```python
from build123d import *

# Parameters (mm, degrees)
SKIZZE1_R                       = 32
SKIZZE1_R_2                     = 22
AUFSATZ_LINEAR_AUSTRAGEN1_DEPTH = 6
SKIZZE4_R                       = 30
SCHNITT_LINEAR_AUSTRAGEN1_DEPTH = 0.1
CUT_EXTRUDE_1_DEPTH             = 264.069580964
DURCHGANGSLOCH_F_R_M41_D        = 4.5
F_5_0_5_DURCHMESSER_BOHRUNG1_D  = 5


with BuildPart() as part:
    # Skizze1 → Aufsatz-Linear austragen1 (new body)
    with BuildSketch(Plane.XY):
        with BuildLine():
            Line((84, 49.943328262), (-234, 49.943328262))
            Line((-234, 49.943328262), (-234, -120.056671738))
            Line((-234, -120.056671738), (-183, -120.056671738))
            Line((-183, -120.056671738), (-183, -118.056671738))
            ThreePointArc((-183, -118.056671738), (-182.414213562, -116.642458175), (-181, -116.056671738))
            Line((-181, -116.056671738), (-170, -116.056671738))
            ThreePointArc((-170, -116.056671738), (-168.585786438, -116.642458175), (-168, -118.056671738))
            Line((-168, -118.056671738), (-168, -120.056671738))
            Line((-168, -120.056671738), (-82.5, -120.056671738))
            Line((-82.5, -120.056671738), (-82.5, -118.056671738))
            ThreePointArc((-82.5, -118.056671738), (-81.914213562, -116.642458175), (-80.5, -116.056671738))
            Line((-80.5, -116.056671738), (-69.5, -116.056671738))
            ThreePointArc((-69.5, -116.056671738), (-68.085786438, -116.642458175), (-67.5, -118.056671738))
            Line((-67.5, -118.056671738), (-67.5, -120.056671738))
            Line((-67.5, -120.056671738), (18, -120.056671738))
            Line((18, -120.056671738), (18, -118.056671738))
            ThreePointArc((18, -118.056671738), (18.585786438, -116.642458175), (20, -116.056671738))
            Line((20, -116.056671738), (31, -116.056671738))
            ThreePointArc((31, -116.056671738), (32.414213562, -116.642458175), (33, -118.056671738))
            Line((33, -118.056671738), (33, -120.056671738))
            Line((33, -120.056671738), (84, -120.056671738))
            Line((84, -120.056671738), (84, 49.943328262))
        make_face()
        with BuildLine():
            Line((-143, -112.556671738), (-103, -112.556671738))
            ThreePointArc((-103, -112.556671738), (-100.5, -115.056671738), (-103, -117.556671738))
            Line((-103, -117.556671738), (-143, -117.556671738))
            ThreePointArc((-143, -117.556671738), (-145.5, -115.056671738), (-143, -112.556671738))
        make_face(mode=Mode.SUBTRACT)
        with BuildLine():
            Line((-7, -117.556671738), (-47, -117.556671738))
            ThreePointArc((-47, -117.556671738), (-49.5, -115.056671738), (-47, -112.556671738))
            Line((-47, -112.556671738), (-7, -112.556671738))
            ThreePointArc((-7, -112.556671738), (-4.5, -115.056671738), (-7, -117.556671738))
        make_face(mode=Mode.SUBTRACT)
        with Locations((-185, -0.056671738)):
            Circle(SKIZZE1_R, mode=Mode.SUBTRACT)
        with Locations((-75, -0.056671738)):
            Circle(SKIZZE1_R_2, mode=Mode.SUBTRACT)
        with Locations((35, -0.056671738)):
            Circle(SKIZZE1_R, mode=Mode.SUBTRACT)
    extrude(amount=AUFSATZ_LINEAR_AUSTRAGEN1_DEPTH)

    # Skizze4 → Schnitt-Linear austragen1 (cut)
    # profile 1 of 2: a face of its own
    with BuildSketch(Plane.XY.offset(6)):
        with BuildLine():
            Line((66, -37.056671738), (4, -37.056671738))
            ThreePointArc((4, -37.056671738), (-0.242640687, -35.299312425), (-2, -31.056671738))
            Line((-2, -31.056671738), (-2, 30.943328262))
            ThreePointArc((-2, 30.943328262), (-0.242640687, 35.185968949), (4, 36.943328262))
            Line((4, 36.943328262), (35, 36.943328262))
            Line((35, 36.943328262), (66, 36.943328262))
            ThreePointArc((66, 36.943328262), (70.242640687, 35.185968949), (72, 30.943328262))
            Line((72, 30.943328262), (72, -31.056671738))
            ThreePointArc((72, -31.056671738), (70.242640687, -35.299312425), (66, -37.056671738))
        make_face()
        with Locations((35, -0.056671738)):
            Circle(SKIZZE4_R, mode=Mode.SUBTRACT)
        with BuildLine():
            Line((64, 22.943328262), (60, 22.943328262))
            ThreePointArc((60, 22.943328262), (57, 25.943328262), (60, 28.943328262))
            Line((60, 28.943328262), (64, 28.943328262))
            ThreePointArc((64, 28.943328262), (67, 25.943328262), (64, 22.943328262))
        make_face(mode=Mode.SUBTRACT)
        with BuildLine():
            Line((10, 28.943328262), (6, 28.943328262))
            ThreePointArc((6, 28.943328262), (3, 25.943328262), (6, 22.943328262))
            Line((6, 22.943328262), (10, 22.943328262))
            ThreePointArc((10, 22.943328262), (13, 25.943328262), (10, 28.943328262))
        make_face(mode=Mode.SUBTRACT)
        with BuildLine():
            Line((10, -29.056671738), (6, -29.056671738))
            ThreePointArc((6, -29.056671738), (3, -26.056671738), (6, -23.056671738))
            Line((6, -23.056671738), (10, -23.056671738))
            ThreePointArc((10, -23.056671738), (13, -26.056671738), (10, -29.056671738))
        make_face(mode=Mode.SUBTRACT)
        with BuildLine():
            Line((60, -29.056671738), (64, -29.056671738))
            ThreePointArc((64, -29.056671738), (67, -26.056671738), (64, -23.056671738))
            Line((64, -23.056671738), (60, -23.056671738))
            ThreePointArc((60, -23.056671738), (57, -26.056671738), (60, -29.056671738))
        make_face(mode=Mode.SUBTRACT)
    # profile 2 of 2: a face of its own
    with BuildSketch(Plane.XY.offset(6)):
        with BuildLine():
            Line((-185, 36.943328262), (-216, 36.943328262))
            ThreePointArc((-216, 36.943328262), (-220.242640687, 35.185968949), (-222, 30.943328262))
            Line((-222, 30.943328262), (-222, -31.056671738))
            ThreePointArc((-222, -31.056671738), (-220.242640687, -35.299312425), (-216, -37.056671738))
            Line((-216, -37.056671738), (-154, -37.056671738))
            ThreePointArc((-154, -37.056671738), (-149.757359313, -35.299312425), (-148, -31.056671738))
            Line((-148, -31.056671738), (-148, 30.943328262))
            ThreePointArc((-148, 30.943328262), (-149.757359313, 35.185968949), (-154, 36.943328262))
            Line((-154, 36.943328262), (-185, 36.943328262))
        make_face()
        with Locations((-185, -0.056671738)):
            Circle(SKIZZE4_R, mode=Mode.SUBTRACT)
        with BuildLine():
            Line((-214, -23.056671738), (-210, -23.056671738))
            ThreePointArc((-210, -23.056671738), (-207, -26.056671738), (-210, -29.056671738))
            Line((-210, -29.056671738), (-214, -29.056671738))
            ThreePointArc((-214, -29.056671738), (-217, -26.056671738), (-214, -23.056671738))
        make_face(mode=Mode.SUBTRACT)
        with BuildLine():
            Line((-210, 28.943328262), (-214, 28.943328262))
            ThreePointArc((-214, 28.943328262), (-217, 25.943328262), (-214, 22.943328262))
            Line((-214, 22.943328262), (-210, 22.943328262))
            ThreePointArc((-210, 22.943328262), (-207, 25.943328262), (-210, 28.943328262))
        make_face(mode=Mode.SUBTRACT)
        with BuildLine():
            Line((-156, -23.056671738), (-160, -23.056671738))
            ThreePointArc((-160, -23.056671738), (-163, -26.056671738), (-160, -29.056671738))
            Line((-160, -29.056671738), (-156, -29.056671738))
            ThreePointArc((-156, -29.056671738), (-153, -26.056671738), (-156, -23.056671738))
        make_face(mode=Mode.SUBTRACT)
        with BuildLine():
            Line((-156, 22.943328262), (-160, 22.943328262))
            ThreePointArc((-160, 22.943328262), (-163, 25.943328262), (-160, 28.943328262))
            Line((-160, 28.943328262), (-156, 28.943328262))
            ThreePointArc((-156, 28.943328262), (-153, 25.943328262), (-156, 22.943328262))
        make_face(mode=Mode.SUBTRACT)
    extrude(amount=-SCHNITT_LINEAR_AUSTRAGEN1_DEPTH, mode=Mode.SUBTRACT)

    # Эскиз2 → Вырез-Вытянуть1 (cut, through all)
    with BuildSketch(Plane.XY.offset(6)):
        with BuildLine():
            Line((-214, -29.056671738), (-210, -29.056671738))
            ThreePointArc((-210, -29.056671738), (-207, -26.056671738), (-210, -23.056671738))
            Line((-210, -23.056671738), (-214, -23.056671738))
            ThreePointArc((-214, -23.056671738), (-217, -26.056671738), (-214, -29.056671738))
        make_face()
        with BuildLine():
            Line((-160, -29.056671738), (-156, -29.056671738))
            ThreePointArc((-156, -29.056671738), (-153, -26.056671738), (-156, -23.056671738))
            Line((-156, -23.056671738), (-160, -23.056671738))
            ThreePointArc((-160, -23.056671738), (-163, -26.056671738), (-160, -29.056671738))
        make_face()
        with BuildLine():
            Line((-156, 28.943328262), (-160, 28.943328262))
            ThreePointArc((-160, 28.943328262), (-163, 25.943328262), (-160, 22.943328262))
            Line((-160, 22.943328262), (-156, 22.943328262))
            ThreePointArc((-156, 22.943328262), (-153, 25.943328262), (-156, 28.943328262))
        make_face()
        with BuildLine():
            Line((-214, 22.943328262), (-210, 22.943328262))
            ThreePointArc((-210, 22.943328262), (-207, 25.943328262), (-210, 28.943328262))
            Line((-210, 28.943328262), (-214, 28.943328262))
            ThreePointArc((-214, 28.943328262), (-217, 25.943328262), (-214, 22.943328262))
        make_face()
        with BuildLine():
            Line((6, 22.943328262), (10, 22.943328262))
            ThreePointArc((10, 22.943328262), (13, 25.943328262), (10, 28.943328262))
            Line((10, 28.943328262), (6, 28.943328262))
            ThreePointArc((6, 28.943328262), (3, 25.943328262), (6, 22.943328262))
        make_face()
        with BuildLine():
            Line((64, 28.943328262), (60, 28.943328262))
            ThreePointArc((60, 28.943328262), (57, 25.943328262), (60, 22.943328262))
            Line((60, 22.943328262), (64, 22.943328262))
            ThreePointArc((64, 22.943328262), (67, 25.943328262), (64, 28.943328262))
        make_face()
        with BuildLine():
            Line((64, -23.056671738), (60, -23.056671738))
            ThreePointArc((60, -23.056671738), (57, -26.056671738), (60, -29.056671738))
            Line((60, -29.056671738), (64, -29.056671738))
            ThreePointArc((64, -29.056671738), (67, -26.056671738), (64, -23.056671738))
        make_face()
        with BuildLine():
            Line((10, -23.056671738), (6, -23.056671738))
            ThreePointArc((6, -23.056671738), (3, -26.056671738), (6, -29.056671738))
            Line((6, -29.056671738), (10, -29.056671738))
            ThreePointArc((10, -29.056671738), (13, -26.056671738), (10, -23.056671738))
        make_face()
    extrude(amount=-CUT_EXTRUDE_1_DEPTH, mode=Mode.SUBTRACT)

    # Durchgangsloch für M41 (through all)
    with Locations(Plane(origin=(0, 0, 0), x_dir=(-1, 0, 0), z_dir=(0, 0, -1))):
        with Locations((75, 28.943328262), (95.506096654, 20.449424917), (104, -0.056671738), (95.506096654, -20.562768392), (75, -29.056671738), (54.493903346, -20.562768392), (46, -0.056671738), (54.493903346, 20.449424917)):
            Hole(DURCHGANGSLOCH_F_R_M41_D / 2)

    # Ø5.0 (5) Durchmesser Bohrung1 (through all)
    with Locations(Plane(origin=(-176.5, -85.056671738, 6), x_dir=(1, 0, 0), z_dir=(0, 0, 1))):
        with Locations((0, 0), (0, 24), (22.5, 24), (45, 24), (45, 0), (22.5, 0), (158, 24), (180.5, 24), (203, 24), (203, 0), (180.5, 0), (158, 0)):
            Hole(F_5_0_5_DURCHMESSER_BOHRUNG1_D / 2)


solid = part.part
```
The listing builds one solid part. Answer for the finished solid, in the listing's coordinates (mm). A direction names the side the tool comes from. Give positions to 0.01 mm unless a question says otherwise; leave off trailing zeros. Order: outer loops, then holes, each group sorted by start corner. A loop starts at its lowest first (then second) coordinate and runs counter-clockwise, first axis right, second up. Notation, with made-up numbers: (68, 0) -> (83, 0) arc R20 ccw to (83, 38) -> close; hole circle Ø7 at (77, 8.5). An arc over 180 degrees is marked (long way). One line per item, written item: value.
1) Find section A-A, the plane y = -6. Determine the outline of the cut face in (x, z).
Reported:
outline: (-234, 0) -> (-216.44, 0) -> (-216.44, 5.9) -> (-222, 5.9) -> (-222, 6) -> (-234, 6) -> close; (-153.56, 0) -> (-96.18, 0) -> (-96.18, 6) -> (-148, 6) -> (-148, 5.9) -> (-153.56, 5.9) -> close; (-53.82, 0) -> (3.56, 0) -> (3.56, 5.9) -> (-2, 5.9) -> (-2, 6) -> (-53.82, 6) -> close; (66.44, 0) -> (84, 0) -> (84, 6) -> (72, 6) -> (72, 5.9) -> (66.44, 5.9) -> close
2) Find section C-C, the plane x = -192.5. Determine the outline of the cut face in (y, z).
Reported:
outline: (-120.06, 0) -> (-31.17, 0) -> (-31.17, 5.9) -> (-37.06, 5.9) -> (-37.06, 6) -> (-120.06, 6) -> close; (31.05, 0) -> (49.94, 0) -> (49.94, 6) -> (36.94, 6) -> (36.94, 5.9) -> (31.05, 5.9) -> close
3) Find section B-B, the plane x = -116. Determine the outline of the cut face in (y, z), plus the area to 3 significant figures.
Reported:
outline: (-120.06, 0) -> (-117.56, 0) -> (-117.56, 6) -> (-120.06, 6) -> close; (-112.56, 0) -> (49.94, 0) -> (49.94, 6) -> (-112.56, 6) -> close
area: 990 mm^2
4) Find section D-D, the plane z = 1.8. Count the separate pieces of the cut face and the enclosed holes in it, plus the area to 3 significant figures.
Reported:
separate pieces: 1
enclosed holes: 33
area: 44,700 mm^2
5) Find the intervals of material crossed by line 1 (Y direction, x = -75, z = 1.5); line 2 (Y direction, x = -46, z = 4.6); line 3 (Y direction, x = -18.5, z = 2.85), in increasing order.
Reported:
line 1: y = -116.06 to -31.31, -26.81 to -22.06, 21.94 to 26.69, 31.19 to 49.94
line 2: y = -120.06 to -117.56, -112.56 to -2.31, 2.19 to 49.94
line 3: y = -120.06 to -117.56, -112.56 to -87.56, -82.56 to -63.56, -58.56 to 49.94
6) A tool of negligible diameter and unlimited length cuts with its end or side. For faces 3 (the cylindrical face through (-163, 26, 3)), 4 (the flat face through (-75, -116.057, 3)), from which of +Z, -Z, +X, -X, +Y, -Y can it reach the whole face along a straight path? Write none if from no direction.
Reported:
face 3: +Z, -Z
face 4: +Z, -Z, -Y
7) Determine the mould class of faces 1 (the flat face through (-27, -112.557, 3)), 2 (the flat face through (-77, -34, 6)) for opening direction X: pulls with the +X half, pulls with the -X half, needs draft (parallel to the pull), parting line crosses it, or undercut.
Reported:
face 1: undercut
face 2: needs draft
